Build history of the part. All positions in model axes, mm. Give positions to 0.01 mm unless a question says otherwise; leave off trailing zeros. Loops run counter-clockwise (first coordinate to the right, second up) from the corner with the lowest first, then second, coordinate; pieces in that order, holes last. Notation, with made-up numbers: (67, 44) -> (100, 44) arc R20 ccw to (100, 60) -> close; hole circle Ø1 at (20, 86). An arc over 180 degrees is marked (long way). Answer as a JSON object with one key per item and string values. Group by question number.
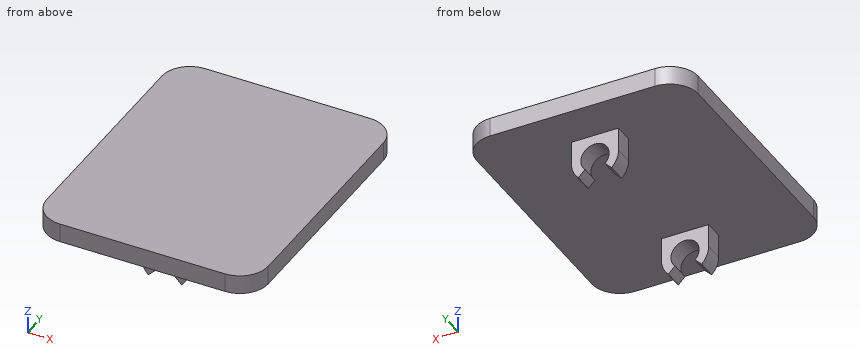
from build123d import *

# Parameters (mm, degrees)
F1_DEPTH = 2
F2_W     = 5
F2_H     = 2
F3_DEPTH = 5
F5_DEPTH = 25


with BuildPart() as f1:
    # F0 (on Top) → F1 (new body)
    with BuildSketch(Plane.XY):
        with BuildLine():
            Line((-8.75, -14.5), (8.75, -14.5))
            ThreePointArc((8.75, -14.5), (10.87132, -13.62132), (11.75, -11.5))
            Line((11.75, -11.5), (11.75, 11.5))
            ThreePointArc((11.75, 11.5), (10.87132, 13.62132), (8.75, 14.5))
            Line((8.75, 14.5), (-8.75, 14.5))
            ThreePointArc((-8.75, 14.5), (-10.87132, 13.62132), (-11.75, 11.5))
            Line((-11.75, 11.5), (-11.75, -11.5))
            ThreePointArc((-11.75, -11.5), (-10.87132, -13.62132), (-8.75, -14.5))
        make_face()
    extrude(amount=F1_DEPTH)

    # F2 (on face) → F3 (join)
    with BuildSketch(Plane(origin=(0, 0, 0), x_dir=(1, 0, 0), z_dir=(0, 0, -1))):
        with Locations((0, 9)):
            Rectangle(F2_W, F2_H)
        with Locations((0, -9)):
            Rectangle(F2_W, F2_H)
    extrude(amount=F3_DEPTH)

    # F4 (on face) → F5 (cut)
    with BuildSketch(Plane.XZ.offset(10)):
        with BuildLine():
            ThreePointArc((2.5, -2.5), (2.309699, -3.456709), (1.767767, -4.267767))
            Line((1.767767, -4.267767), (1.06066, -3.56066))
            ThreePointArc((1.06066, -3.56066), (0, -1), (-1.06066, -3.56066))
            Line((-1.06066, -3.56066), (-1.767767, -4.267767))
            ThreePointArc((-1.767767, -4.267767), (-2.309699, -3.456709), (-2.5, -2.5))
            Line((-2.5, -2.5), (-2.5, -5))
            Line((-2.5, -5), (2.5, -5))
            Line((2.5, -5), (2.5, -2.5))
        make_face()
        Polygon((3.523229, -2.854811), (2.5, -2.5), (2.5, -5), (-2.5, -5), (-2.5, -2.5), (-3.529894, -2.823659), (-4.289252, -6.509164), (2.408858, -5.650775), (4.006271, -4.421826), align=None)
    extrude(amount=-F5_DEPTH, mode=Mode.SUBTRACT)


solid = f1.part
(1) Saw through at A-A on x = 0. List the corners of the cut face in (y, z).
(2) Saw through at C-C on y = 4. List the corners of the cut face in (x, z).
(3) Saw through at B-B on z = -1.75. List the corners of the cut face in (x, y).
(4) Pin check, flat tips, straight feed: pin 1 (1.3 mm diameter, centred on x = 1, z = -1.5, fed in from -Y); pin 2 (3.5 mm diameter, centred on x = 0, z = -2, fed in from +Y); pin 3 (1.6 mm diameter, centred on y = -8.5, z = -1.5, fed in from +X); pin 4 (1.5 mm diameter, centred on y = 11, z = -2.5, fed in from -X). Stop position of each tip, or through.
(5) Saw through at D-D on x = -3. List the corners of the cut face in (y, z), plus the area to 3 significant figures.
(6) Probe line 1 along X through (y, z) = (-9.15, -2.5); line 2 along Z through (x, y) = (6.75, -9.5); line 3 along Z through (x, y) = (0.5, -8.5). List the from-to ranges inside material, lowest first. Write a range as [from, to].
Calculated:
{
 "1": {"outline": "(-14.5, 0) -> (-10, 0) -> (-10, -1) -> (-8, -1) -> (-8, 0) -> (8, 0) -> (8, -1) -> (10, -1) -> (10, 0) -> (14.5, 0) -> (14.5, 2) -> (-14.5, 2) -> close"},
 "2": {"outline": "(-11.75, 0) -> (11.75, 0) -> (11.75, 2) -> (-11.75, 2) -> close"},
 "3": {"outline": "(-2.5, -10) -> (-1.3, -10) -> (-1.3, -8) -> (-2.5, -8) -> close; (-2.5, 8) -> (-1.3, 8) -> (-1.3, 10) -> (-2.5, 10) -> close; (1.3, -10) -> (2.5, -10) -> (2.5, -8) -> (1.3, -8) -> close; (1.3, 8) -> (2.5, 8) -> (2.5, 10) -> (1.3, 10) -> close"},
 "4": {"pin 1": "stops at y = -10", "pin 2": "stops at y = 10", "pin 3": "stops at x = 2.5", "pin 4": "passes through"},
 "5": {"outline": "(-14.5, 0) -> (14.5, 0) -> (14.5, 2) -> (-14.5, 2) -> close", "area": "58.0 mm^2"},
 "6": {"line 1": "x = [-2.5, -1.5], [1.5, 2.5]", "line 2": "z = [0, 2]", "line 3": "z = [-1.09, 2]"}
}
